Geometry: see drawing. Coordinates: mm, zero at the bounding-box minimum. A direction names the side the tool comes from. Coordinates: 2 decimals unless noted, no trailing zeros. Write each loop counter-clockwise with the first axis right and the second up, starting at its lowest first coordinate (ties: lowest second). Pieces come first, ordered by that corner, then holes. Notation, with made-up numbers: (10.25, 45.5) - (41.25, 45.5) arc R11 ccw to (41.25, 66.5) - close; hole circle Ø10 at (30.25, -23.5). An arc over 180 degrees is marked (long way). Use a Markdown table: item, result. Add a question column.
Q1. Set-up query: the marked faces 1, 2, 3, 4 and 5. Return all of +Z, -Z, +X, -X, +Y, -Y with unobstructed straight access to the full face (end or side cutting, diameter ignored); none if empty.
Q2. Pin query (flat end, axial travel): P1, Ø1.5, axis at x = 1, z = 4.5, coming from the +Y side; P2, Ø0.8, axis at x = 4.5, z = 8, coming from the -Y side (1 decimal); P3, Ø1.9, axis at y = 18.5, z = 7.5, coming from the -X side; P4, Ø1, axis at x = 18, y = 19.5, coming from the -Z side. Return the tip coordinate at first contact, or that it passes through.
Q3. Section query A-A (y = 11.25). Return the cut outline in (x, z), then the cut area to 3 significant figures.
Q4. Mould query, pull axis Y, two halves, no side actions, for the marked faces 6, 7 and 8. Classes: released by +Y, released by -Y, zero draft, split by the parting line, or undercut.
Q5. Section query D-D (x = 19.5). Return the cut outline in (y, z).
Q6. Material intervals for probe 1 along Y at (x, z) = (20.75, 6.5); probe 2 along X at (y, z) = (7.5, 2.25) (1 decimal); probe 3 along X at (y, z) = (9.25, 2), sorted ascending. Write a range as from..to.
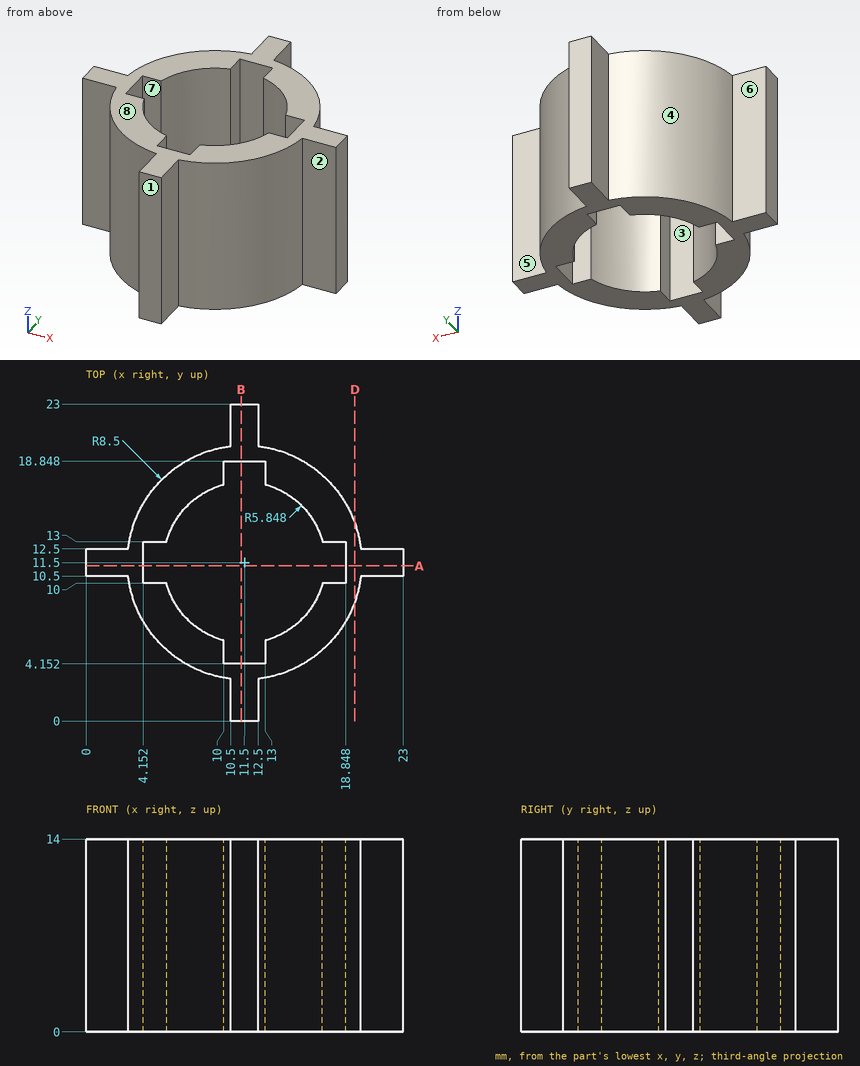
Values follow:
| question | item | result |
|---|---|---|
| 1 | face 1 | +Z, -Z, +X, -X, -Y |
| 1 | face 2 | +Z, -Z, +X, -Y |
| 1 | face 3 | +Z, -Z |
| 1 | face 4 | +Z, -Z, -X, +Y |
| 1 | face 5 | +Z, -Z, +X, +Y |
| 2 | P1 | y = 12.5 |
| 2 | P2 | y = 6.1 |
| 2 | P3 | x = 5.53 |
| 2 | P4 | through |
| 3 | outline | (0, 0) - (4.15, 0) - (4.15, 14) - (0, 14) - close; (18.85, 0) - (23, 0) - (23, 14) - (18.85, 14) - close |
| 3 | area | 116 mm2 |
| 4 | face 6 | released by +Y |
| 4 | face 7 | undercut |
| 4 | face 8 | zero draft |
| 5 | outline | (8.63, 0) - (14.37, 0) - (14.37, 14) - (8.63, 14) - close |
| 6 | probe 1 | 10.5..12.5 |
| 6 | probe 2 | 4..7.2, 15.8..19 |
| 6 | probe 3 | 3.3..6.1, 16.9..19.7 |
